Design review of the part built by this model. Coordinates are the model's own, in mm. A direction names the side the tool comes from. Give positions to 0.01 mm unless a question says otherwise; leave off trailing zeros. Loops run counter-clockwise (first coordinate to the right, second up) from the corner with the lowest first, then second, coordinate; pieces in that order, holes last. Notation, with made-up numbers: (69, -24.75) -> (90, -24.75) arc R28 ccw to (90, 11.25) -> close; hole circle Ø9 at (-4.5, 72.5). An arc over 180 degrees is marked (long way). Answer in a Markdown table with one row per item. Add a question column.
(1) For faces 1 (the cylindrical face through (-1.5, 0.07, 1.97)), 2 (the flat face through (-2, -2, 0.1)), list the 3-axis set-ups (+Z, -Z, +X, -X, +Y, -Y) from which the entire face can be reached by the end or side of a thin tool; tool diameter is ignored.
(2) Consider section D-D on y = -2.5. Write out the cut boundary in (x, z), then the cut area to 3 significant figures.
(3) Consider section A-A on y = 0. Write out the cut boundary in (x, z).
(4) Draft analysis for pull direction X (two halves, no side actions). For faces 3 (the flat face through (2, -2, 3.9)), 4 (the cylindrical face through (-0.867, -3.905, 1.972)), state which applies: +X half, -X half, draft (parallel to the pull), parting line (faces both ways), or undercut.
(5) Consider section C-C on z = 0.9. Write out the cut boundary in (x, y).
(6) For line 1 (Y direction, x = 0, z = 1.55); line 2 (X direction, y = 1, z = 1.4), list the stretches that pass through material, from the lowest coordinate up.
(7) For pin 1 (1 mm diameter, centred on x = -3, z = 1.5, fed in from +Y); pin 2 (1 mm diameter, centred on x = 2.5, z = 2, fed in from +Y); pin 3 (2 mm diameter, centred on x = 1.5, z = 1, fed in from -Y), all flat-tipped, find the tip position at first contact; note any pin that passes through.
from build123d import *

# Parameters (mm, degrees)
SKETCH1_R           = 4
SKETCH1_R_2         = 1.5
BOSS_EXTRUDE1_DEPTH = 4
SKETCH2_R           = 3.7
SKETCH2_R_2         = 1.975178003
CUT_EXTRUDE1_DEPTH  = 0.1
SKETCH3_R           = 3.7
SKETCH3_R_2         = 1.975178003
CUT_EXTRUDE2_DEPTH  = 0.1


with BuildPart() as part:
    # Sketch1 → Boss-Extrude1 (new body)
    with BuildSketch(Plane.XY):
        Circle(SKETCH1_R)
        Circle(SKETCH1_R_2, mode=Mode.SUBTRACT)
    extrude(amount=BOSS_EXTRUDE1_DEPTH)

    # Sketch2 → Cut-Extrude1 (cut)
    with BuildSketch(Plane.XY.offset(4)):
        Circle(SKETCH2_R)
        Circle(SKETCH2_R_2, mode=Mode.SUBTRACT)
    extrude(amount=-CUT_EXTRUDE1_DEPTH, mode=Mode.SUBTRACT)

    # Sketch3 → Cut-Extrude2 (cut)
    with BuildSketch(Plane(origin=(0, 0, 0), x_dir=(-1, 0, 0), z_dir=(0, 0, -1))):
        Circle(SKETCH3_R)
        Circle(SKETCH3_R_2, mode=Mode.SUBTRACT)
    extrude(amount=-CUT_EXTRUDE2_DEPTH, mode=Mode.SUBTRACT)


solid = part.part
Values follow:
| question | item | result |
|---|---|---|
| 1 | face 1 | +Z, -Z |
| 1 | face 2 | -Z |
| 2 | outline | (-3.12, 0) -> (-2.73, 0) -> (-2.73, 0.1) -> (2.73, 0.1) -> (2.73, 0) -> (3.12, 0) -> (3.12, 4) -> (2.73, 4) -> (2.73, 3.9) -> (-2.73, 3.9) -> (-2.73, 4) -> (-3.12, 4) -> close |
| 2 | area | 23.9 mm2 |
| 3 | outline | (-4, 0) -> (-3.7, 0) -> (-3.7, 0.1) -> (-1.98, 0.1) -> (-1.98, 0) -> (-1.5, 0) -> (-1.5, 4) -> (-1.98, 4) -> (-1.98, 3.9) -> (-3.7, 3.9) -> (-3.7, 4) -> (-4, 4) -> close; (1.5, 0) -> (1.98, 0) -> (1.98, 0.1) -> (3.7, 0.1) -> (3.7, 0) -> (4, 0) -> (4, 4) -> (3.7, 4) -> (3.7, 3.9) -> (1.98, 3.9) -> (1.98, 4) -> (1.5, 4) -> close |
| 4 | face 3 | undercut |
| 4 | face 4 | parting line |
| 5 | outline | circle Ø8 at (0, 0); hole circle Ø3 at (0, 0) |
| 6 | line 1 | -4 to -1.5, 1.5 to 4 |
| 6 | line 2 | -3.87 to -1.12, 1.12 to 3.87 |
| 7 | pin 1 | y = 3.12 |
| 7 | pin 2 | y = 3.46 |
| 7 | pin 3 | y = -3.97 |
